The model under review builds one solid part; all positions refer to its coordinate system, in mm. Round coordinates to 2 decimals unless told otherwise and drop trailing zeros. Write each loop counter-clockwise with the first axis right and the second up, starting at its lowest first coordinate (ties: lowest second). Pieces come first, ordered by that corner, then holes. Notation, with made-up numbers: (5.5, 64.5) -> (61.5, 64.5) arc R21 cw to (61.5, 74.5) -> close; hole circle Ø3 at (10.5, 24.5). An arc over 180 degrees is marked (long way). Use CSV: the item, a comma, the result in double quotes. Start each with the question number.
1) For pin 1 Ø3.5 at (x, z) = (0, 15) entering from +Y, flat-tipped, find the tip position at first contact; note if it passes through.
2) Take a section at A-A, the plane z = -15. Give the boundary of the cut face in (x, y), then the cut area to 3 significant figures.
3) Mouldability with a two-part tool opening along X and no side actions: class faces 1 (the face through (0, 3, -30)), 2 (the face through (-7.5, 3, 0)), 3 (the face through (7.5, 3, 0)), 4 (the face through (-0.676, 3.057, -12.854)) as released by +X, released by -X, zero draft, split by the parting line, or undercut.
4) Wall thickness on probe 1 along Z at (x, y) = (0, 2.25); probe 2 along X at (y, z) = (5.25, -15); probe 3 along Z at (x, y) = (-1, 3): over which ranges is each line inside the solid? List them lowest first. Write a range as [from, to].
5) Take a section at C-C, the plane x = 0. Give the boundary of the cut face in (y, z), then the cut area to 3 significant figures.
6) Take a section at B-B, the plane y = 1. Give the boundary of the cut face in (x, z).
Autodesk Inventor part; units mm, degrees
ref_plane "YZ Plane" through (0, 0, 0) normal (1, 0, 0) x (0, 1, 0)
ref_plane "XZ Plane" through (0, 0, 0) normal (0, 1, 0) x (-1, 0, 0)
ref_plane "XY Plane" through (0, 0, 0) normal (0, 0, 1) x (1, 0, 0)
sketch "Sketch1" plane through (0, 0, 0) normal (0, 1, 0) x (-1, 0, 0)
  line L0 (-7.5, -30) -> (7.5, -30)
  line L1 (7.5, -30) -> (7.5, 30)
  line L2 (7.5, 30) -> (-7.5, 30)
  line L3 (-7.5, 30) -> (-7.5, -30)
  line L4 (-7.5, -30) -> (7.5, 30) construction
  line L5 (7.5, -30) -> (-7.5, 30) construction
  point P0 (0, 0)
  dimension "d0" = 15
  dimension "d1" = 60
extrude "Extrusion1" add sketch "Sketch1" along normal blind 6.2
sketch "Sketch2" plane through (0, 6.2, 0) normal (0, 1, 0) x (1, 0, 0)
  line L0 (-7.5, -30) -> (7.5, -30)
  line L1 (7.5, 30) -> (-7.5, 30)
  point P0 (0, 0)
  point P1 (0, -15)
  point P2 (0, 15)
  point P3 (0, -30)
  dimension "d4" = 15
  dimension "d5" = 15
hole "Hole1" at (0, 6.2, 15) at (0, 6.2, -15) direction (0, -1, 0) diameter 4.5 end through all
properties part number "Ajuste vertical"
Values found:
1,pin 1,"through"
2,outline,"(-7.5, 0) -> (-2.25, 0) -> (-2.25, 6.2) -> (-7.5, 6.2) -> close; (2.25, 0) -> (7.5, 0) -> (7.5, 6.2) -> (2.25, 6.2) -> close"
2,area,"65.1 mm²"
3,face 1,"zero draft"
3,face 2,"released by -X"
3,face 3,"released by +X"
3,face 4,"undercut"
4,probe 1,"[-30, -17.25], [-12.75, 12.75], [17.25, 30]"
4,probe 2,"[-7.5, -2.25], [2.25, 7.5]"
4,probe 3,"[-30, -17.02], [-12.98, 12.98], [17.02, 30]"
5,outline,"(0, -30) -> (6.2, -30) -> (6.2, -17.25) -> (0, -17.25) -> close; (0, -12.75) -> (6.2, -12.75) -> (6.2, 12.75) -> (0, 12.75) -> close; (0, 17.25) -> (6.2, 17.25) -> (6.2, 30) -> (0, 30) -> close"
5,area,"316 mm²"
6,outline,"(-7.5, -30) -> (7.5, -30) -> (7.5, 30) -> (-7.5, 30) -> close; hole circle Ø4.5 at (0, -15); hole circle Ø4.5 at (0, 15)"
